from build123d import *

# Parameters (mm, degrees)
SKETCH_1_R      = 1
EXTRUDE_1_DEPTH = 8


with BuildPart() as part:
    # 草圖1 → 填料-伸長1 (new body)
    with BuildSketch(Plane(origin=(0, 0, 0), x_dir=(1, 0, 0), z_dir=(0, 1, 0))):
        with BuildLine():
            Line((0, 0), (0, 12.2))
            Line((0, 12.2), (-22.5, 12.2))
            Line((-22.5, 12.2), (-22.5, 0))
            Line((-22.5, 0), (-27.124303732, 0))
            ThreePointArc((-27.124303732, 0), (-31.398520886, 0.462060812), (-35.475243216, 1.826893228))
            Line((-35.475243216, 1.826893228), (-55.835093948, 11.182689323))
            ThreePointArc((-55.835093948, 11.182689323), (-56.953793919, 13.427421715), (-55, 15))
            Line((-55, 15), (5, 15))
            ThreePointArc((5, 15), (12.5, 7.5), (5, 0))
            Line((5, 0), (0, 0))
        make_face()
        with Locations(Location((-25, 6.1, 0), (0, 0, 270))):
            Circle(SKETCH_1_R, mode=Mode.SUBTRACT)
        with Locations(Location((2.5, 6.1, 0), (0, 0, 270))):
            Circle(SKETCH_1_R, mode=Mode.SUBTRACT)
    extrude(amount=EXTRUDE_1_DEPTH)


solid = part.part
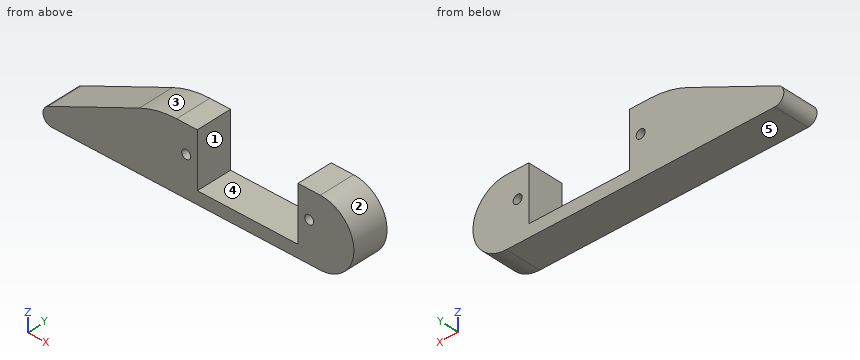
Can you work these out from the model? Positions are in its coordinate system, mm. Face numbers are marked on the shaded views. A direction names the side the tool comes from. Give positions to 0.01 mm unless a question says otherwise; leave off trailing zeros. Loops run counter-clockwise (first coordinate to the right, second up) from the corner with the lowest first, then second, coordinate; pieces in that order, holes last. Notation, with made-up numbers: (-34.75, 47.5) -> (21.25, 47.5) arc R24 cw to (21.25, 68.5) -> close; hole circle Ø2 at (1, 62.5). An arc over 180 degrees is marked (long way). Use one line per item in the form item = value.
1) If we section it at D-D (z = -6.5): Please give me the cut outline in (x, y), plus the area to 3 significant figures.
Answers:
outline = (-45.64, 0) -> (-25.92, 0) -> (-25.92, 8) -> (-45.64, 8) -> close; (-24.08, 0) -> (-22.5, 0) -> (-22.5, 8) -> (-24.08, 8) -> close; (0, 0) -> (1.58, 0) -> (1.58, 8) -> (0, 8) -> close; (3.42, 0) -> (12.43, 0) -> (12.43, 8) -> (3.42, 8) -> close
area = 255 mm²
2) Will these pins go through, and if not, where does the flat tip stop? pin 1 (2.5 mm diameter, centred on x = -13.5, y = 4, fed in from +Z); pin 2 (1.5 mm diameter, centred on y = 6, z = -3, fed in from +X); pin 3 (1 mm diameter, centred on x = -49.5, y = 1, fed in from +Z).
Answers:
pin_1 = -12.2
pin_2 = 11.5
pin_3 = -8.04
3) I need wall thicknesses on line 1 along X through (y, z) = (4.5, -6.1); line 2 along Z through (x, y) = (-5, 3); line 3 along X through (y, z) = (6.75, -2). Which ranges of each line are inside material? Lowest first, please.
Answers:
line_1 = -44.77 to -26, -24 to -22.5, 0 to 1.5, 3.5 to 12.37
line_2 = -15 to -12.2
line_3 = -35.85 to -22.5, 0 to 10.1
4) We'd pull the mould along X, two halves only. Please class the marked faces 1, 2 and 3: released by +X, released by -X, zero draft, split by the parting line, or undercut.
Answers:
face_1 = undercut
face_2 = released by +X
face_3 = released by -X
5) If we section it at C-C (z = -0.75): Please give me the cut outline in (x, y), plus the area to 3 significant figures.
Answers:
outline = (-32.55, 0) -> (-22.5, 0) -> (-22.5, 8) -> (-32.55, 8) -> close; (0, 0) -> (8.27, 0) -> (8.27, 8) -> (0, 8) -> close
area = 147 mm²
6) If we section it at A-A (x = 2.5): Please give me the cut outline in (y, z).
Answers:
outline = (0, -15) -> (8, -15) -> (8, -7.1) -> (0, -7.1) -> close; (0, -5.1) -> (8, -5.1) -> (8, 0) -> (0, 0) -> close
7) If we section it at B-B (y = 4.5): Please give me the cut outline in (x, z).
Answers:
outline = (-55.84, -11.18) arc R2 ccw to (-55, -15) -> (5, -15) arc R7.5 ccw to (5, 0) -> (0, 0) -> (0, -12.2) -> (-22.5, -12.2) -> (-22.5, 0) -> (-27.12, 0) arc R20 ccw to (-35.48, -1.83) -> close; hole circle Ø2 at (-25, -6.1); hole circle Ø2 at (2.5, -6.1)
8) For the marked faces 4 and 5, which set-ups out of +Z, -Z, +X, -X, +Y, -Y let a thin tool reach every point of the face, with its end or its side?
Answers:
face_4 = +Z, +Y, -Y
face_5 = -Z, +X, -X, +Y, -Y
